```python
from build123d import *

# Parameters (mm, degrees)
MODEL_R             = 1.6
BOSS_EXTRUDE1_DEPTH = 3


with BuildPart() as part:
    # Model → Boss-Extrude1 (new body)
    with BuildSketch(Plane.XY):
        with BuildLine():
            Line((295.043822464, 218.133419689), (281.478366665, 218.133419689))
            Line((281.478366665, 218.133419689), (281.478366665, 158.133416479))
            ThreePointArc((281.478366665, 158.133416479), (282.064153103, 156.719202917), (283.478366665, 156.133416479))
            Line((283.478366665, 156.133416479), (332.478366665, 156.133416479))
            ThreePointArc((332.478366665, 156.133416479), (333.892580227, 156.719202917), (334.478366665, 158.133416479))
            Line((334.478366665, 158.133416479), (334.478366665, 210.48904049))
            Line((334.478366665, 210.48904049), (328.509839464, 218.133396046))
            Line((328.509839464, 218.133396046), (323.975870464, 218.133396046))
            ThreePointArc((323.975870464, 218.133396046), (323.725870171, 218.066408731), (323.542857332, 217.883395759))
            ThreePointArc((323.542857332, 217.883395759), (322.756291514, 217.779840053), (322.859842674, 218.566406469))
            ThreePointArc((322.859842674, 218.566406469), (323.042854191, 218.749419176), (323.109840891, 218.999418473))
            Line((323.109840891, 218.999418473), (323.109840891, 220.633447473))
            ThreePointArc((323.109840891, 220.633447473), (322.963394282, 220.987000863), (322.609840891, 221.133447473))
            Line((322.609840891, 221.133447473), (317.609843891, 221.133447473))
            ThreePointArc((317.609843891, 221.133447473), (317.256293472, 220.987003641), (317.109844085, 220.633455522))
            Line((317.109844085, 220.633455522), (317.109844085, 218.999428522))
            ThreePointArc((317.109844085, 218.999428522), (317.176831025, 218.749428628), (317.35984329, 218.566415765))
            ThreePointArc((317.35984329, 218.566415765), (317.463395273, 217.779850295), (316.676829874, 217.883402813))
            ThreePointArc((316.676829874, 217.883402813), (316.49381775, 218.066414713), (316.243818787, 218.133402112))
            Line((316.243818787, 218.133402112), (311.109839721, 218.133402112))
            Line((311.109839721, 218.133402112), (311.109839721, 215.333404229))
            Line((311.109839721, 215.333404229), (312.534860417, 215.333404229))
            Line((312.534860417, 215.333404229), (312.534860417, 211.133417963))
            Line((312.534860417, 211.133417963), (311.109850498, 211.133417963))
            Line((311.109850498, 211.133417963), (311.109850498, 208.133417963))
            Line((311.109850498, 208.133417963), (307.909850498, 208.133417963))
            Line((307.909850498, 208.133417963), (307.909850498, 211.133417963))
            Line((307.909850498, 211.133417963), (306.634859186, 211.133417963))
            Line((306.634859186, 211.133417963), (306.634859186, 215.333417963))
            Line((306.634859186, 215.333417963), (307.909850498, 215.333417963))
            Line((307.909850498, 215.333417963), (307.909850498, 218.133417963))
            Line((307.909850498, 218.133417963), (302.775874676, 218.133417963))
            ThreePointArc((302.775874676, 218.133417963), (302.525874676, 218.066430665), (302.342861974, 217.883417963))
            ThreePointArc((302.342861974, 217.883417963), (301.556296087, 217.779862777), (301.659847768, 218.566429125))
            ThreePointArc((301.659847768, 218.566429125), (301.842859406, 218.749441711), (301.909846272, 218.999440963))
            Line((301.909846272, 218.999440963), (301.909846272, 220.633469963))
            ThreePointArc((301.909846272, 220.633469963), (301.763399662, 220.987023354), (301.409846272, 221.133469963))
            Line((301.409846272, 221.133469963), (296.409849272, 221.133469963))
            ThreePointArc((296.409849272, 221.133469963), (296.056295709, 220.987026085), (295.909846369, 220.633474785))
            Line((295.909846369, 220.633474785), (295.909846369, 218.999447785))
            ThreePointArc((295.909846369, 218.999447785), (295.976833795, 218.749448021), (296.159846417, 218.566435514))
            ThreePointArc((296.159846417, 218.566435514), (296.263399931, 217.779870247), (295.47683433, 217.883421233))
            ThreePointArc((295.47683433, 217.883421233), (295.293821724, 218.066432851), (295.043822464, 218.133419689))
        make_face()
        with Locations((286.989833469, 186.133406309)):
            Circle(MODEL_R, mode=Mode.SUBTRACT)
        with BuildLine():
            Line((325.609838719, 176.133405309), (325.609838719, 186.133405309))
            ThreePointArc((325.609838719, 186.133405309), (314.509838719, 197.233405309), (303.409838719, 186.133405309))
            Line((303.409838719, 186.133405309), (303.409838719, 176.133405309))
            ThreePointArc((303.409838719, 176.133405309), (314.509838719, 165.033405309), (325.609838719, 176.133405309))
        make_face(mode=Mode.SUBTRACT)
        with BuildLine():
            Line((331.609838719, 160.633405309), (331.609838719, 170.636460624))
            ThreePointArc((331.609838719, 170.636460624), (330.009838719, 172.236460624), (328.409838719, 170.636460624))
            Line((328.409838719, 170.636460624), (328.409838719, 160.633405309))
            ThreePointArc((328.409838719, 160.633405309), (330.009838719, 159.033405309), (331.609838719, 160.633405309))
        make_face(mode=Mode.SUBTRACT)
        with BuildLine():
            Line((331.609838719, 201.633405309), (331.609838719, 191.630349994))
            ThreePointArc((331.609838719, 191.630349994), (330.009838719, 190.030349994), (328.409838719, 191.630349994))
            Line((328.409838719, 191.630349994), (328.409838719, 201.633405309))
            ThreePointArc((328.409838719, 201.633405309), (330.009838719, 203.233405309), (331.609838719, 201.633405309))
        make_face(mode=Mode.SUBTRACT)
        with BuildLine():
            Line((297.409838719, 160.633405309), (297.409838719, 170.636460624))
            ThreePointArc((297.409838719, 170.636460624), (299.009838719, 172.236460624), (300.609838719, 170.636460624))
            Line((300.609838719, 170.636460624), (300.609838719, 160.633405309))
            ThreePointArc((300.609838719, 160.633405309), (299.009838719, 159.033405309), (297.409838719, 160.633405309))
        make_face(mode=Mode.SUBTRACT)
        with BuildLine():
            Line((297.409838719, 201.633405309), (297.409838719, 191.630349994))
            ThreePointArc((297.409838719, 191.630349994), (299.009838719, 190.030349994), (300.609838719, 191.630349994))
            Line((300.609838719, 191.630349994), (300.609838719, 201.633405309))
            ThreePointArc((300.609838719, 201.633405309), (299.009838719, 203.233405309), (297.409838719, 201.633405309))
        make_face(mode=Mode.SUBTRACT)
        with BuildLine():
            Line((288.639792166, 173.001169926), (288.639792166, 177.469119926))
            ThreePointArc((288.639792166, 177.469119926), (288.706781285, 177.719120392), (288.889796147, 177.902132238))
            ThreePointArc((288.889796147, 177.902132238), (288.993345727, 178.688698026), (288.206780642, 178.585143097))
            ThreePointArc((288.206780642, 178.585143097), (288.023768466, 178.402130146), (287.773768823, 178.335142269))
            Line((287.773768823, 178.335142269), (286.205898823, 178.335142269))
            ThreePointArc((286.205898823, 178.335142269), (285.955899571, 178.402129135), (285.772886985, 178.585140772))
            ThreePointArc((285.772886985, 178.585140772), (284.986321396, 178.688691846), (285.089874823, 177.902126567))
            ThreePointArc((285.089874823, 177.902126567), (285.272887674, 177.719113607), (285.339874823, 177.469113269))
            Line((285.339874823, 177.469113269), (285.339874823, 173.001163269))
            ThreePointArc((285.339874823, 173.001163269), (285.272887957, 172.751164017), (285.089876319, 172.568151431))
            ThreePointArc((285.089876319, 172.568151431), (284.986324638, 171.781585083), (285.772890525, 171.885140269))
            ThreePointArc((285.772890525, 171.885140269), (285.955903052, 172.06815287), (286.205902823, 172.135140269))
            Line((286.205902823, 172.135140269), (287.773770823, 172.135140269))
            ThreePointArc((287.773770823, 172.135140269), (288.023770203, 172.068153881), (288.206783139, 171.885142594))
            ThreePointArc((288.206783139, 171.885142594), (288.993349685, 171.781592418), (288.889792994, 172.568158106))
            ThreePointArc((288.889792994, 172.568158106), (288.706780043, 172.751170283), (288.639792166, 173.001169926))
        make_face(mode=Mode.SUBTRACT)
        with BuildLine():
            Line((285.339870115, 199.26564477), (285.339870115, 194.79769477))
            ThreePointArc((285.339870115, 194.79769477), (285.272883249, 194.547695518), (285.089871611, 194.364682932))
            ThreePointArc((285.089871611, 194.364682932), (284.986320538, 193.578117343), (285.772885817, 193.68167077))
            ThreePointArc((285.772885817, 193.68167077), (285.955898344, 193.864683371), (286.205898115, 193.93167077))
            Line((286.205898115, 193.93167077), (287.773766115, 193.93167077))
            ThreePointArc((287.773766115, 193.93167077), (288.023765495, 193.864684382), (288.206778431, 193.681673095))
            ThreePointArc((288.206778431, 193.681673095), (288.993344977, 193.578122919), (288.889788286, 194.364688607))
            ThreePointArc((288.889788286, 194.364688607), (288.706775085, 194.547701217), (288.639787458, 194.797701427))
            Line((288.639787458, 194.797701427), (288.639787458, 199.265650427))
            ThreePointArc((288.639787458, 199.265650427), (288.70677658, 199.515650897), (288.889791447, 199.698662743))
            ThreePointArc((288.889791447, 199.698662743), (288.993341016, 200.485228531), (288.206775935, 200.381673598))
            ThreePointArc((288.206775935, 200.381673598), (288.023763758, 200.198660647), (287.773764115, 200.13167277))
            Line((287.773764115, 200.13167277), (286.205894115, 200.13167277))
            ThreePointArc((286.205894115, 200.13167277), (285.955894863, 200.198659636), (285.772882277, 200.381671273))
            ThreePointArc((285.772882277, 200.381671273), (284.986316688, 200.485222347), (285.089870115, 199.698657068))
            ThreePointArc((285.089870115, 199.698657068), (285.272882716, 199.515644541), (285.339870115, 199.26564477))
        make_face(mode=Mode.SUBTRACT)
    extrude(amount=BOSS_EXTRUDE1_DEPTH)


solid = part.part
```
Design review of the part built by this model. Coordinates are the model's own, in mm. A direction names the side the tool comes from. Give positions to 0.01 mm unless a question says otherwise; leave off trailing zeros. Write each loop counter-clockwise with the first axis right and the second up, starting at its lowest first coordinate (ties: lowest second). Pieces come first, ordered by that corner, then holes. Notation, with made-up numbers: (-10, 55.5) - (13, 55.5) arc R17 cw to (13, 59.5) - close; hole circle Ø5 at (36.5, -5.75). An arc over 180 degrees is marked (long way). Return JSON: item names as keys, results as strings. Group by question number.
(1) We need section C-C, the plane y = 188.5. Give the boundary of the cut face in (x, z), then the cut area to 3 significant figures.
(2) We need section D-D, the plane z = 1. Give the number of separate pieces and of enclosed holes in the cut face, then the cut area to 3 significant figures.
(3) We need section B-B, the plane x = 298.5. Give the boundary of the cut face in (y, z).
(4) Mouldability with a two-part tool opening along Y and no side actions: class faces 4 (the flat face through (334.478, 184, 1)), 5 (the flat face through (288.64, 175, 1)), 6 (the cylindrical face through (282.049, 156.735, 1.479)), 7 (the flat face through (314, 218.133, 1)) as +Y half, -Y half, draft (parallel to the pull), parting line (faces both ways), or undercut.
(5) We need section A-A, the plane x = 321. Give the boundary of the cut face in (y, z), then the cut area to 3 significant figures.
(6) To check wall thickness, follow probe 1 along X at (y, z) = (198.5, 2.5); probe 2 along X at (y, z) = (177.5, 1.75); probe 3 along X at (y, z) = (173, 2.65). State the ranges of each line that lie inside material, in increasing order.
(7) Machinability: for faces 1 (the flat face through (308, 156.133, 1)), 2 (the flat face through (307.91, 210, 1)), 3 (the flat face through (312.535, 213, 1)), which of the approach directions +Z, -Z, +X, -X, +Y, -Y give a long, thin tool a straight path to every point of the face, cutting with its end or side? Answer none if there is none.
(8) Insertion check: pin 1 (1.6 mm diameter, centred on x = 285.34, y = 193.93, fed in from -Z); pin 2 (1 mm diameter, centred on x = 311, z = 2, fed in from +Y); pin 3 (1.4 mm diameter, centred on y = 217, z = 2, fed in from +X); pin 4 (1.5 mm diameter, centred on y = 213, z = 2, fed in from +X). Each pin has a flat end and moves straight along its axis. Give the tip position at first contact, or say it passes through.
Reported:
{
 "1": {"outline": "(281.48, 0) - (303.67, 0) - (303.67, 3) - (281.48, 3) - close; (325.35, 0) - (334.48, 0) - (334.48, 3) - (325.35, 3) - close", "area": "93.9 mm2"},
 "2": {"separate pieces": "1", "enclosed holes": "8", "area": "2,430 mm2"},
 "3": {"outline": "(156.13, 0) - (159.12, 0) - (159.12, 3) - (156.13, 3) - close; (172.15, 0) - (190.11, 0) - (190.11, 3) - (172.15, 3) - close; (203.15, 0) - (221.13, 0) - (221.13, 3) - (203.15, 3) - close"},
 "4": {"face 4": "draft", "face 5": "undercut", "face 6": "-Y half", "face 7": "+Y half"},
 "5": {"outline": "(156.13, 0) - (167.13, 0) - (167.13, 3) - (156.13, 3) - close; (195.14, 0) - (221.13, 0) - (221.13, 3) - (195.14, 3) - close", "area": "111 mm2"},
 "6": {"probe 1": "x = 281.48 to 285.34, 288.64 to 297.41, 300.61 to 328.41, 331.61 to 334.48", "probe 2": "x = 281.48 to 285.34, 288.64 to 303.41, 325.61 to 334.48", "probe 3": "x = 281.48 to 285.34, 288.64 to 303.86, 325.16 to 334.48"},
 "7": {"face 1": "+Z, -Z, +X, -X, -Y", "face 2": "+Z, -Z, +Y", "face 3": "+Z, -Z"},
 "8": {"pin 1": "stops at z = 0", "pin 2": "stops at y = 218.13", "pin 3": "stops at x = 329.94", "pin 4": "stops at x = 333.1"}
}
